```python
from build123d import *

# Parameters (mm, degrees)
BOSS_EXTRUDE1_DEPTH = 9
BOSS_EXTRUDE2_START = -8
SKETCH3_R           = 1
BOSS_EXTRUDE2_DEPTH = 1
FILLET3_R           = 3


with BuildPart() as part:
    # Sketch1 → Boss-Extrude1 (new, symmetric)
    with BuildSketch(Plane.XY):
        with BuildLine():
            Line((18.897662626, 0), (-18.897662626, 0))
            ThreePointArc((-18.897662626, 0), (-19.863071357, -0.248433278), (-20.588640432, -0.932014017))
            Line((-20.588640432, -0.932014017), (-25.052631579, -8))
            Line((-25.052631579, -8), (-24.207142676, -8.533992991))
            Line((-24.207142676, -8.533992991), (-19.743151529, -1.466007009))
            ThreePointArc((-19.743151529, -1.466007009), (-19.380366991, -1.124216639), (-18.897662626, -1))
            Line((-18.897662626, -1), (18.897662626, -1))
            ThreePointArc((18.897662626, -1), (19.380366991, -1.124216639), (19.743151529, -1.466007009))
            Line((19.743151529, -1.466007009), (26.101879518, -11.533992991))
            Line((26.101879518, -11.533992991), (26.947368421, -11))
            Line((26.947368421, -11), (20.588640432, -0.932014017))
            ThreePointArc((20.588640432, -0.932014017), (19.863071357, -0.248433278), (18.897662626, 0))
        make_face()
    extrude(amount=BOSS_EXTRUDE1_DEPTH, both=True)

    # Sketch3 → Boss-Extrude2 (add)
    with BuildSketch(Plane.XY.offset(BOSS_EXTRUDE2_START)):
        with BuildLine():
            Line((0, 0), (10.848900056, 7.635533222))
            ThreePointArc((10.848900056, 7.635533222), (12.385192628, 7.962556149), (13.683904275, 7.07910444))
            Line((13.683904275, 7.07910444), (16.271066443, 3.403151108))
            ThreePointArc((16.271066443, 3.403151108), (16.813414859, 2.3083729), (17, 1.10095122))
            Line((17, 1.10095122), (17, 0))
            Line((17, 0), (0, 0))
        make_face()
        with Locations((12, 6)):
            Circle(SKETCH3_R, mode=Mode.SUBTRACT)
    boss_extrude2 = extrude(amount=BOSS_EXTRUDE2_DEPTH)

    # Mirror1: Boss-Extrude2 across plane
    add(boss_extrude2.mirror(Plane.XY))

    # Fillet3
    fillet3_edges = [part.edges().sort_by_distance(p)[0] for p in [
        (26.52462397, -11.266996496, 9),
        (-24.629887127, -8.266996496, -9),
        (26.52462397, -11.266996496, -9),
        (-24.629887127, -8.266996496, 9),
    ]]
    fillet(fillet3_edges, radius=FILLET3_R)


solid = part.part
```
Here's how the part is built. I have some questions about the finished solid (model axes, mm). A direction names the side the tool comes from. Coordinates: 2 decimals unless noted, no trailing zeros. Write each loop counter-clockwise with the first axis right and the second up, starting at its lowest first coordinate (ties: lowest second). Pieces come first, ordered by that corner, then holes. Notation, with made-up numbers: (24, 17) - (57, 17) arc R24 cw to (57, 37) - close; hole circle Ø4 at (37, 5.25). An arc over 180 degrees is marked (long way). One line per item, written item: value.
1) I need wall thicknesses on line 1 along Y through (x, z) = (12, -7.75); line 2 along Y through (x, z) = (-18, -6.25); line 3 along X through (y, z) = (-2.75, -7.5). Which ranges of each line are inside material? Lowest first, please.
Model answer:
line 1: y = -1 to 5, 7 to 8
line 2: y = -1 to 0
line 3: x = -21.74 to -20.55, 20.55 to 21.74
2) Suppose I cut it at C-C on y = -3.25. Write out the boundary of the cut face in (x, z).
Model answer:
outline: (-22.05, -9) - (-20.87, -9) - (-20.87, 9) - (-22.05, 9) - close; (20.87, -9) - (22.05, -9) - (22.05, 9) - (20.87, 9) - close
3) Suppose I cut it at A-A on x = 12. Write out the boundary of the cut face in (y, z).
Model answer:
outline: (-1, -9) - (0, -9) - (0, -8) - (5, -8) - (5, -7) - (0, -7) - (0, 7) - (5, 7) - (5, 8) - (0, 8) - (0, 9) - (-1, 9) - close; (7, -8) - (8, -8) - (8, -7) - (7, -7) - close; (7, 7) - (8, 7) - (8, 8) - (7, 8) - close
4) Suppose I cut it at B-B on z = -3.5. Write out the boundary of the cut face in (x, y), and give its area (3 significant figures).
Model answer:
outline: (-25.05, -8) - (-24.21, -8.53) - (-19.74, -1.47) arc R1 cw to (-18.9, -1) - (18.9, -1) arc R1 cw to (19.74, -1.47) - (26.1, -11.53) - (26.95, -11) - (20.59, -0.93) arc R2 ccw to (18.9, 0) - (-18.9, 0) arc R2 ccw to (-20.59, -0.93) - close
area: 61.1 mm²
5) We'd pull the mould along X, two halves only. Please class faces 4 (the flat face through (22.88, -6.43, 0.13)), 5 (the flat face through (5.349, 3.764, 7.507)), 6 (the cylindrical face through (16.81, 2.32, 7.51)): pulls with the +X half, pulls with the -X half, needs draft (parallel to the pull), parting line crosses it, or undercut.
Model answer:
face 4: undercut
face 5: pulls with the -X half
face 6: pulls with the +X half
6) Suppose I cut it at D-D on y = 6. Write out the boundary of the cut face in (x, z), and give its area (3 significant figures).
Model answer:
outline: (8.53, -8) - (11, -8) - (11, -7) - (8.53, -7) - close; (8.53, 7) - (11, 7) - (11, 8) - (8.53, 8) - close; (13, -8) - (14.44, -8) - (14.44, -7) - (13, -7) - close; (13, 7) - (14.44, 7) - (14.44, 8) - (13, 8) - close
area: 7.84 mm²
7) I'm going to push flat-ended pins straight in: P1, Ø2.5, axis at x = 8, y = 3.5, coming from the +Z side; P2, Ø0.5, axis at y = 0.5, z = 7.5, coming from the +X side; P3, Ø1, axis at x = 16, z = 5, coming from the +Y side; P4, Ø1.2, axis at x = 12, y = 6, coming from the +Z side. Where does each tip first touch, or does it pass through?
Model answer:
P1: stops at z = 8
P2: stops at x = 17
P3: stops at y = 0
P4: passes through
8) On a 3-axis mill with a long thin cutter (end or side, diameter ignored), from which of +Z, -Z, +X, -X, +Y, -Y can I reach the whole of each face in a straight line? I mean faces 1 (the flat face through (11, 3, 8)), 2 (the flat face through (11, 3, 7)), 3 (the flat face through (0, -1, 0)). Say none if no direction works.
Model answer:
face 1: +Z, +X, -X, +Y
face 2: +X, -X, +Y
face 3: +Z, -Z, -Y
